For this review, take the finished solid that the model builds, in its own axes (mm). Give positions to 0.01 mm unless a question says otherwise; leave off trailing zeros. Write each loop counter-clockwise with the first axis right and the second up, starting at its lowest first coordinate (ties: lowest second). Pieces come first, ordered by that corner, then holes.
1) Wall thickness on line 1 along Y through (x, z) = (90, 4.25); line 2 along Y through (x, z) = (-31, 2.75): over which ranges is each line inside the solid? List them lowest first.
2) We need section A-A on x = 60. Give the boundary of the cut face in (y, z).
3) We need section B-B on z = 4. Give the number of separate pieces and of enclosed holes in the cut face, and give its area (3 significant figures).
4) Draft analysis for pull direction X (two halves, no side actions). For faces 1 (the face through (150, -1, 5)), 2 (the face through (-63, -21, 5)), 3 (the face through (-2, 1, 0)), 4 (the face through (-85.12, 26.08, 4.93)), state which applies: pulls with the +X half, pulls with the -X half, needs draft (parallel to the pull), parting line crosses it, or undercut.
Autodesk Inventor part; units mm, degrees
ref_plane "YZ Plane" through (0, 0, 0) normal (1, 0, 0) x (0, 1, 0)
ref_plane "XZ Plane" through (0, 0, 0) normal (0, 1, 0) x (-1, 0, 0)
ref_plane "XY Plane" through (0, 0, 0) normal (0, 0, 1) x (1, 0, 0)
sketch "Skizze1" plane through (0, 0, 0) normal (0, 0, 1) x (1, 0, 0)
  line L0 (-150, -50) -> (150, -50)
  line L1 (150, -50) -> (150, 50)
  line L2 (150, 50) -> (-150, 50)
  line L3 (-150, 50) -> (-150, -50)
  line L4 (-210, 0) -> (210, 0)
  line L5 (0, -70) -> (0, 70)
  point P0 (0, 0)
  dimension "d0" = 300
  dimension "d1" = 100
extrude "Extrusion1" add sketch "Skizze1" along normal blind 10
sketch "Skizze2" plane through (0, 0, 10) normal (0, 0, 1) x (1, 0, 0)
  line L0 (-210, 0) -> (210, 0)
  line L1 (0, -70) -> (0, 70)
  line L2 (-150, 50) -> (-150, -50)
  point P0 (0, 0)
  point P1 (-120, -25)
  dimension "d4" = 25
  dimension "d5" = 30
hole "Bohrung1" at (-120, -25, 10) direction (0, 0, -1) diameter 10 end through all
pattern_linear "Rechteckige Anordnung1" count 9 spacing 30 along (1, 0, 0) count 2 spacing 50 along (0, 1, 0) of "Bohrung1"
properties part number "Lochplatte"
Results list:
1. line 1: y = -50 to -30, -20 to 20, 30 to 50
1. line 2: y = -50 to -29.9, -20.1 to 20.1, 29.9 to 50
2. outline: (-50, 0) - (-30, 0) - (-30, 10) - (-50, 10) - close; (-20, 0) - (20, 0) - (20, 10) - (-20, 10) - close; (30, 0) - (50, 0) - (50, 10) - (30, 10) - close
3. separate pieces: 1
3. enclosed holes: 18
3. area: 28,600 mm2
4. face 1: pulls with the +X half
4. face 2: undercut
4. face 3: needs draft
4. face 4: undercut
